Geometry check sheet. Reference: the model listing, model coordinates, mm. Face numbers are marked on the shaded views. A direction names the side the tool comes from. Coordinates: 2 decimals unless noted, no trailing zeros. Order: outer loops, then holes, each group sorted by start corner. A loop starts at its lowest first (then second) coordinate and runs counter-clockwise, first axis right, second up. Notation, with made-up numbers: (29, -15) -> (77, -15) arc R31 cw to (77, 10) -> close; hole circle Ø2 at (54.5, 80). An arc over 180 degrees is marked (long way). Answer in a Markdown table with one row per item. Add a question column.
```python
from build123d import *

# Parameters (mm, degrees)
SKETCH1_W            = 50
SKETCH1_H            = 40
BODY_DEPTH           = 12
FILLETBODY_R         = 3
SKETCH41_R           = 1.575
CHANNEL1_DEPTH       = 57
SKETCH42_R           = 2.575
INLET_DEPTH          = 5
SKETCH43_R           = 2.575
OUTLET_DEPTH         = 5
SKETCH44_R           = 15
WINDOW_DEPTH         = 5.5
SKETCH45_W           = 16
SKETCH45_H           = 10
FLOWCH_DEPTH         = 5.575
SKETCH46_W           = 10
SKETCH46_H           = 10
WINDOW_HOLE_DEPTH    = 16
SKETCH49_R           = 1.5
FIXHOLES_DEPTH       = 2
GASKET_DEPTH         = 1
SKETCH3_R            = 1.5
BOLT_HOLE_DEPTH      = 10
BOLT_HOLE_DEPTH_BACK = 31


with BuildPart() as part:
    # Sketch1 → Body (new body)
    with BuildSketch(Plane(origin=(0, 0, 0), x_dir=(1, 0, 0), z_dir=(0, 1, 0))):
        Rectangle(SKETCH1_W, SKETCH1_H)
    extrude(amount=BODY_DEPTH)

    # FilletBody
    filletbody_edges = [part.edges().sort_by_distance(p)[0] for p in [
        (-25, 6, -20),
        (25, 6, -20),
        (25, 6, 20),
        (-25, 6, 20),
    ]]
    fillet(filletbody_edges, radius=FILLETBODY_R)

    # Sketch41 → Channel1 (cut)
    with BuildSketch(Plane.ZY.offset(25)):
        with Locations((0, 4)):
            Circle(SKETCH41_R)
    extrude(amount=-CHANNEL1_DEPTH, mode=Mode.SUBTRACT)

    # Sketch42 → Inlet (cut)
    with BuildSketch(Plane.ZY.offset(25)):
        with Locations((0, 4)):
            Circle(SKETCH42_R)
    extrude(amount=-INLET_DEPTH, mode=Mode.SUBTRACT)

    # Sketch43 → Outlet (cut)
    with BuildSketch(Plane(origin=(25, 0, 0), x_dir=(0, 0, -1), z_dir=(1, 0, 0))):
        with Locations((0, 4)):
            Circle(SKETCH43_R)
    extrude(amount=-OUTLET_DEPTH, mode=Mode.SUBTRACT)

    # Sketch44 → Window (cut)
    with BuildSketch(Plane(origin=(0, 12, 0), x_dir=(1, 0, 0), z_dir=(0, 1, 0))):
        Circle(SKETCH44_R)
    extrude(amount=-WINDOW_DEPTH, mode=Mode.SUBTRACT)

    # Sketch45 → FlowCh (cut)
    with BuildSketch(Plane.XZ):
        Rectangle(SKETCH45_W, SKETCH45_H)
    extrude(amount=-FLOWCH_DEPTH, mode=Mode.SUBTRACT)

    # Sketch46 → Window_hole (cut)
    with BuildSketch(Plane(origin=(0, 6.5, 0), x_dir=(1, 0, 0), z_dir=(0, 1, 0))):
        Rectangle(SKETCH46_W, SKETCH46_H)
    extrude(amount=-WINDOW_HOLE_DEPTH, mode=Mode.SUBTRACT)

    # Sketch49 → FixHoles (cut)
    with BuildSketch(Plane(origin=(0, 6.5, 0), x_dir=(1, 0, 0), z_dir=(0, 1, 0))):
        with Locations((0, 11)):
            Circle(SKETCH49_R)
        with Locations((0, -11)):
            Circle(SKETCH49_R)
    extrude(amount=-FIXHOLES_DEPTH, mode=Mode.SUBTRACT)

    # Sketch50 → Gasket (cut)
    with BuildSketch(Plane.XZ):
        with BuildLine():
            ThreePointArc((8, 11), (12.242640687, 9.242640687), (14, 5))
            Line((14, 5), (14, -5))
            ThreePointArc((14, -5), (12.242640687, -9.242640687), (8, -11))
            Line((8, -11), (-8, -11))
            ThreePointArc((-8, -11), (-12.242640687, -9.242640687), (-14, -5))
            Line((-14, -5), (-14, 5))
            ThreePointArc((-14, 5), (-12.242640687, 9.242640687), (-8, 11))
            Line((-8, 11), (8, 11))
        make_face()
        with BuildLine():
            Line((-8, -7), (8, -7))
            ThreePointArc((8, -7), (9.414213562, -6.414213562), (10, -5))
            Line((10, -5), (10, 5))
            ThreePointArc((10, 5), (9.414213562, 6.414213562), (8, 7))
            Line((8, 7), (-8, 7))
            ThreePointArc((-8, 7), (-9.414213562, 6.414213562), (-10, 5))
            Line((-10, 5), (-10, -5))
            ThreePointArc((-10, -5), (-9.414213562, -6.414213562), (-8, -7))
        make_face(mode=Mode.SUBTRACT)
    extrude(amount=-GASKET_DEPTH, mode=Mode.SUBTRACT)

    # Sketch3 → Bolt_hole (cut, two sides)
    with BuildSketch(Plane(origin=(0, 12, 0), x_dir=(1, 0, 0), z_dir=(0, 1, 0))) as bolt_hole_sk:
        with Locations((-17.5, 12.5)):
            Circle(SKETCH3_R)
        with Locations((17.5, 12.5)):
            Circle(SKETCH3_R)
        with Locations((17.5, -12.5)):
            Circle(SKETCH3_R)
        with Locations((-17.5, -12.5)):
            Circle(SKETCH3_R)
    extrude(amount=BOLT_HOLE_DEPTH, mode=Mode.SUBTRACT)
    extrude(bolt_hole_sk.sketch, amount=-BOLT_HOLE_DEPTH_BACK, mode=Mode.SUBTRACT)


solid = part.part
```
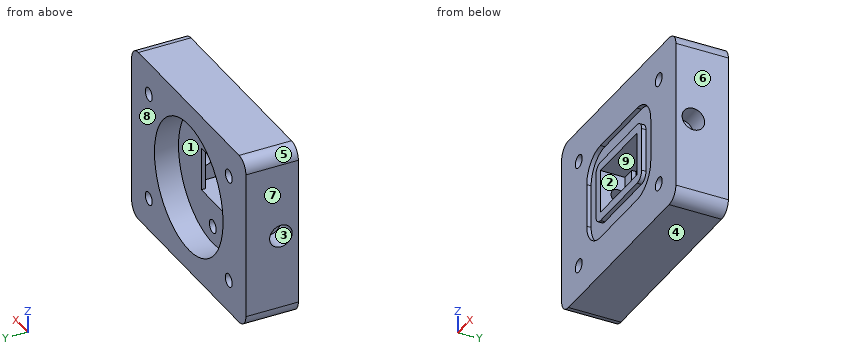
(1) Cross-section at C-C (y = 10.25). Enter the section's corners in (x, z), plus the area to 3 significant figures.
(2) Access from +Z, -Z, +X, -X, +Y, -Y to the whole of each face (thin tool, end or side, straight path). Record for the marked faces 1, 2, 3, 4 and 5.
(3) Cross-section at A-A (x = 17.5). Enter the section's corners in (y, z) (3 decimals), plus the area to 3 significant figures.
(4) Cross-section at D-D (x = -9). Enter the section's corners in (y, z) (3 decimals), plus the area to 3 significant figures.
(5) Scan lines: line 1 along Z through (x, y) = (-17.5, 9); line 2 along X through (y, z) = (2.25, 3); line 3 along Z through (x, y) = (0, 5.75). Record each from-to range of solid material in increasing order.
(6) Go/stop test with flat-tipped pins: P1, Ø4, axis at x = 13.5, z = -1.5, coming from the -Y side; P2, Ø9, axis at x = 4, z = 3.5, coming from the +Y side; P3, Ø1.5, axis at x = 0, z = 11, coming from the +Y side; P4, Ø4, axis at y = 3.5, z = 0, coming from the -X side. Record where each tip stops, or that it passes through.
(7) Mould release check, pull along X, two halves, no side actions. Record for the marked faces 6, 7, 8 and 9: +X half, -X half, draft (parallel to the pull), parting line (faces both ways), or undercut.
(8) Cross-section at B-B (x = 0). Enter the section's corners in (y, z), plus the area to 3 significant figures.
Checks:
| question | item | result |
|---|---|---|
| 1 | outline | (-25, -17) arc R3 ccw to (-22, -20) -> (22, -20) arc R3 ccw to (25, -17) -> (25, 17) arc R3 ccw to (22, 20) -> (-22, 20) arc R3 ccw to (-25, 17) -> close; hole circle Ø3 at (-17.5, -12.5); hole circle Ø3 at (-17.5, 12.5); hole circle Ø30 at (0, 0); hole circle Ø3 at (17.5, -12.5); hole circle Ø3 at (17.5, 12.5) |
| 1 | area | 1,260 mm² |
| 2 | face 1 | +Y |
| 2 | face 2 | -Y |
| 2 | face 3 | -X |
| 2 | face 4 | -Z, +X, -X, +Y, -Y |
| 2 | face 5 | +Z, -X, +Y, -Y |
| 3 | outline | (0, -20) -> (12, -20) -> (12, -14) -> (0, -14) -> close; (0, -11) -> (12, -11) -> (12, 11) -> (0, 11) -> close; (0, 14) -> (12, 14) -> (12, 20) -> (0, 20) -> close; hole circle Ø3.15 at (4, 0) |
| 3 | area | 400 mm² |
| 4 | outline | (0, -20) -> (12, -20) -> (12, -12) -> (6.5, -12) -> (6.5, 12) -> (12, 12) -> (12, 20) -> (0, 20) -> (0, 10.916) -> (1, 10.916) -> (1, 6.732) -> (0, 6.732) -> (0, -6.732) -> (1, -6.732) -> (1, -10.916) -> (0, -10.916) -> close; hole circle Ø3.15 at (4, 0) |
| 4 | area | 332 mm² |
| 5 | line 1 | -20 to -14, -11 to 11, 14 to 20 |
| 5 | line 2 | -25 to -8, 8 to 25 |
| 5 | line 3 | -20 to -12.5, -9.5 to -5, 5 to 9.5, 12.5 to 20 |
| 6 | P1 | y = 0 |
| 6 | P2 | y = 6.5 |
| 6 | P3 | y = 4.5 |
| 6 | P4 | x = -20 |
| 7 | face 6 | +X half |
| 7 | face 7 | -X half |
| 7 | face 8 | draft |
| 7 | face 9 | undercut |
| 8 | outline | (0, -20) -> (12, -20) -> (12, -15) -> (6.5, -15) -> (6.5, -12.5) -> (4.5, -12.5) -> (4.5, -9.5) -> (6.5, -9.5) -> (6.5, -5) -> (0, -5) -> (0, -7) -> (1, -7) -> (1, -11) -> (0, -11) -> close; (0, 5) -> (6.5, 5) -> (6.5, 9.5) -> (4.5, 9.5) -> (4.5, 12.5) -> (6.5, 12.5) -> (6.5, 15) -> (12, 15) -> (12, 20) -> (0, 20) -> (0, 11) -> (1, 11) -> (1, 7) -> (0, 7) -> close |
| 8 | area | 230 mm² |
